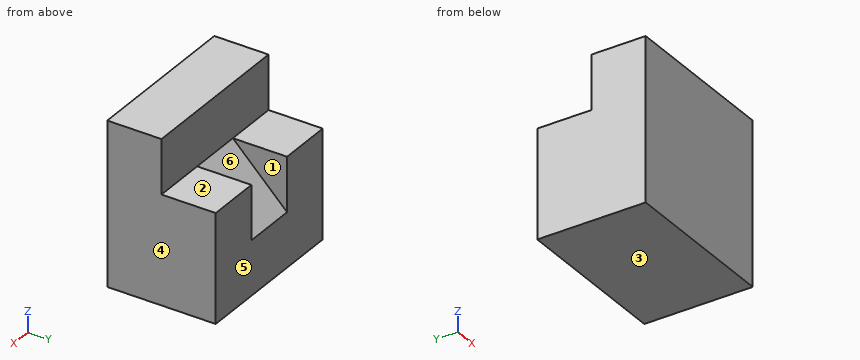
from build123d import *

# Parameters (mm, degrees)
SKETCH10_W              = 60
SKETCH10_H              = 60
BOSS_EXTRUDE6_DEPTH     = 40
SKETCH12_W              = 60
SKETCH12_H              = 20
CUT_EXTRUDE4_DEPTH      = 20
CUT_EXTRUDE7_DEPTH      = 79.102496759
CUT_EXTRUDE7_DEPTH_BACK = 79.102496759
SKETCH26_W              = 20
SKETCH26_H              = 20
BOSS_EXTRUDE8_DEPTH     = 20
SKETCH30_W              = 20
SKETCH30_H              = 20
BOSS_EXTRUDE10_DEPTH    = 20


with BuildPart() as part:
    # Sketch10 → Boss-Extrude6 (new body)
    with BuildSketch(Plane(origin=(0, 0, 0), x_dir=(1, 0, 0), z_dir=(0, 1, 0))):
        Rectangle(SKETCH10_W, SKETCH10_H)
    extrude(amount=BOSS_EXTRUDE6_DEPTH)

    # Sketch12 → Cut-Extrude4 (cut)
    with BuildSketch(Plane.XY.offset(30)):
        with Locations((0, 30)):
            Rectangle(SKETCH12_W, SKETCH12_H)
    extrude(amount=-CUT_EXTRUDE4_DEPTH, mode=Mode.SUBTRACT)

    # Sketch25 → Cut-Extrude7 (cut, two sides: drawn at the far end of the back side and taken through both)
    with BuildSketch(Plane(origin=(30, 0, 0), x_dir=(0, 0, -1), z_dir=(1, 0, 0)).offset(-CUT_EXTRUDE7_DEPTH_BACK)):
        Polygon((-10, 40), (-10, 20), (10, 40), align=None)
    extrude(amount=CUT_EXTRUDE7_DEPTH + CUT_EXTRUDE7_DEPTH_BACK, mode=Mode.SUBTRACT)

    # Sketch26 → Boss-Extrude8 (add)
    with BuildSketch(Plane(origin=(0, 20, 0), x_dir=(1, 0, 0), z_dir=(0, 1, 0))):
        with Locations((-20, 0)):
            Rectangle(SKETCH26_W, SKETCH26_H)
    extrude(amount=BOSS_EXTRUDE8_DEPTH)

    # Sketch30 → Boss-Extrude10 (add)
    with BuildSketch(Plane(origin=(0, 20, 0), x_dir=(1, 0, 0), z_dir=(0, 1, 0))):
        with Locations((20, 0)):
            Rectangle(SKETCH30_W, SKETCH30_H)
    extrude(amount=BOSS_EXTRUDE10_DEPTH)


solid = part.part
For this review, take the finished solid that the model builds, in its own axes (mm). Face numbers are marked on the shaded views. A direction names the side the tool comes from. Give positions to 0.01 mm unless a question says otherwise; leave off trailing zeros. Loops run counter-clockwise (first coordinate to the right, second up) from the corner with the lowest first, then second, coordinate; pieces in that order, holes last. Notation, with made-up numbers: M 81,-0.5 L 112,-0.5 A27 cw 112,31.5 Z; hole C -6,80 d2. An arc over 180 degrees is marked long. Put each result on its own line as item: value. Start each with the question number.
(1) For pin 1 (6 mm diameter, centred on x = -16.5, y = 32.5, fed in from +Z); pin 2 (16 mm diameter, centred on x = 7, z = 20.5, fed in from +Y); pin 3 (6 mm diameter, centred on x = -3.5, z = -1.5, fed in from +Y), all flat-tipped, find the tip position at first contact; note any pin that passes through.
(2) Wall thickness on L1, parallel to Z at x = -17.5, y = 38.5; L2, parallel to Y at x = 10, z = 25; L3, parallel to Z at x = -0.5, y = 26.5: over which ranges is each line inside the solid? List them lowest first.
(3) The part is to be moulded in two halves that separate along X. For the marked faces 4, 5 and 6, say which applies: +X half, -X half, draft (parallel to the pull), parting line (faces both ways), or undercut.
(4) Add section B-B, the plane z = 7. Write out the cut boundary in (x, y).
(5) Add section D-D, the plane x = -18.5. Write out the cut boundary in (y, z).
(6) Add section A-A, the plane y = 21. Write out the cut boundary in (x, z), then the cut area to 3 significant figures.
(7) Machinability: for the marked faces 1, 2 and 3, which of the approach directions +Z, -Z, +X, -X, +Y, -Y give a long, thin tool a straight path to every point of the face, cutting with its end or side? Answer none if there is none.
(8) Add section C-C, the plane x = 3.5. Write out the cut boundary in (y, z).
Result:
1. pin 1: stops at z = 10
1. pin 2: stops at y = 20
1. pin 3: stops at y = 34.5
2. L1: z = -30 to 10
2. L2: y = 0 to 20
2. L3: z = -30 to 3.5
3. face 4: +X half
3. face 5: draft
3. face 6: undercut
4. outline: M -30,0 L 30,0 L 30,40 L 10,40 L 10,23 L -10,23 L -10,40 L -30,40 Z
5. outline: M 0,-30 L 40,-30 L 40,10 L 20,10 L 20,30 L 0,30 Z
6. outline: M -30,-30 L 30,-30 L 30,10 L 10,10 L 10,9 L -10,9 L -10,10 L -30,10 Z
6. area: 2,380 mm^2
7. face 1: +Z, +Y
7. face 2: +Z, +X, -X, +Y
7. face 3: -Z, +X, -X, +Y, -Y
8. outline: M 0,-30 L 40,-30 L 40,-10 L 20,10 L 20,30 L 0,30 Z
